Input: part model. Units: mm. Frame: model coordinates. A direction names the side the tool comes from. Round coordinates to 2 decimals unless told otherwise and drop trailing zeros. Order: outer loops, then holes, each group sorted by start corner. A loop starts at its lowest first (then second) coordinate and runs counter-clockwise, first axis right, second up. Notation, with made-up numbers: M -2.5,30 L 41.5,30 A22 ccw 41.5,62 Z; hole C 79,71 d11. An arc over 180 degrees is marked long. One line per question, with ' | ' between items.
```python
from build123d import *

# Parameters (mm, degrees)
F1_DEPTH = 800
F2_W     = 720
F2_H     = 100
F3_DEPTH = 1140.001


with BuildPart() as f1:
    # F0 (on Front) → F1 (new body)
    with BuildSketch(Plane.XZ):
        Polygon((0, 1050), (0, 0), (40, 0), (40, 100), (930, 100), (930, 0), (970, 0), (970, 850), (80, 1050), (80, 1650), (280, 1800), (280, 2100), (-170, 2100), (-170, 1800), (30, 1650), (30, 1050), align=None)
    extrude(amount=F1_DEPTH)

    # F2 (on face) → F3 (cut, through all)
    with BuildSketch(Plane.YZ.offset(970)):
        with Locations((-400, 50)):
            Rectangle(F2_W, F2_H)
        Polygon((-1182.620752, 1232.519794), (-800, 1050), (-600, 1050), (-600, 1650), (-800, 1650), (-800, 2165.248656), (-400.054373, 2171.843762), (-400.054373, 1650), (-500, 1650), (-500, 1050), (130.563885, 1050), (1207.751429, 1992.828178), (48.128108, 2661.814022), (-1305.009472, 2532.382298), align=None)
    extrude(amount=-F3_DEPTH, mode=Mode.SUBTRACT)


solid = f1.part
```
Item 1: Section query B-B, the plane z = 154. Return loops of the section in (x, y).
Report:
outline: M 0,-800 L 970,-800 L 970,0 L 0,0 Z
Item 2: Mould query, pull axis X, two halves, no side actions, for faces 1 (the flat face through (-170, -597, 1952)), 2 (the flat face through (41, -394, 1050)), 3 (the flat face through (930, -20, 51)). Classes: +X half, -X half, draft (parallel to the pull), parting line (faces both ways), or undercut.
Report:
face 1: -X half | face 2: draft | face 3: undercut
Item 3: Section query C-C, the plane y = -321. Return loops of the section in (x, z), plus the area to 4 significant figures.
Report:
outline: M 0,100 L 970,100 L 970,850 L 80,1050 L 0,1050 Z | area: 832,500 mm²
Item 4: Section query D-D, the plane x = 340.5. Return loops of the section in (y, z).
Report:
outline: M -800,100 L 0,100 L 0,991.46 L -800,991.46 Z
Item 5: Line query: line 1 along X through (y, z) = (-733, 195); line 2 along X through (y, z) = (-480, 1872); line 3 along Y through (x, z) = (-0.5, 1710.5). Output: solid intervals per line, ascending. Write a range as from..to.
Report:
line 1: 0..970 | line 2: -170..280 | line 3: -800..-400.05
Item 6: Section query A-A, the plane y = -632. Return loops of the section in (x, z).
Report:
outline: M -170,1800 L 30,1650 L 80,1650 L 280,1800 L 280,2100 L -170,2100 Z; M 0,100 L 970,100 L 970,850 L 80,1050 L 0,1050 Z
Item 7: First-contact query: pin 1 (6 mm diameter, centred on x = 159, y = -426.5, fed in from -Z); pin 2 (2 mm diameter, centred on y = -316.5, z = 266, fed in from -X). Flat tips, straight axial feed; report the tip coordinate or a pass-through.
Report:
pin 1: z = 100 | pin 2: x = 0
Item 8: Access query for faces 4 (the flat face through (40, -20, 49)), 5 (the flat face through (55, -500, 1354)), 6 (the flat face through (280, -597, 1948)). Directions: +Z, -Z, +X, -X, +Y, -Y. A direction counts if a zero-diameter tool reaches every point of the face in a straight line with its end or side. Return the directions, or none.
Report:
face 4: -Z, +Y, -Y | face 5: +X, -X, +Y | face 6: +Z, +X, +Y, -Y
